from build123d import *

# Parameters (mm, degrees)
BOSS_EXTRU_1_DEPTH      = 3
ENL_V_MAT_EXTRU_1_REACH = 5
ESQUISSE3_R             = 1.75
ESQUISSE4_W             = 52.83
ESQUISSE4_H             = 19.81
BOSS_EXTRU_2_DEPTH      = 2
ESQUISSE6_W             = 6.35
ESQUISSE6_H             = 19.81
BOSS_EXTRU_3_DEPTH      = 9.74
ENL_V_START             = -6
ESQUISSE5_R             = 2.286
ENL_V_MAT_EXTRU_2_DEPTH = 16.74
ESQUISSE7_R             = 4
ENL_V_MAT_EXTRU_3_DEPTH = 6
ESQUISSE8_W             = 1
ESQUISSE8_H             = 2
ENL_V_MAT_EXTRU_4_DEPTH = 53.83
ESQUISSE9_W             = 10.19
ESQUISSE9_H             = 1
ENL_V_MAT_EXTRU_5_DEPTH = 32.415
CONG_1_R                = 2.54
CONG_2_R                = 2.54


with BuildPart() as part:
    # Esquisse2 → Boss.-Extru.1 (new body)
    with BuildSketch(Plane(origin=(0, 0, 0), x_dir=(1, 0, 0), z_dir=(0, 1, 0))):
        with BuildLine():
            Line((-4.999130413, 19.906752432), (-4.999130413, -20.093247568))
            ThreePointArc((-4.999130413, -20.093247568), (0.046625811, -24.999782599), (5, -20))
            Line((5, -20), (5, 20))
            ThreePointArc((5, 20), (-0.046625811, 24.999782599), (-4.999130413, 19.906752432))
        make_face()
    extrude(amount=BOSS_EXTRU_1_DEPTH)

    # Esquisse3 → Enlèv. mat.-Extru.1 (cut, up to next)
    with BuildSketch(Plane(origin=(0, 3, 0), x_dir=(1, 0, 0), z_dir=(0, 1, 0)), mode=Mode.PRIVATE) as enl_v_mat_extru_1_sk1:
        with Locations((0, 20)):
            Circle(ESQUISSE3_R)
    enl_v_mat_extru_1_tool1 = extrude(enl_v_mat_extru_1_sk1.sketch, amount=-ENL_V_MAT_EXTRU_1_REACH, mode=Mode.PRIVATE) & part.part
    add(enl_v_mat_extru_1_tool1.solids().sort_by_distance((0, 3, -20))[0], mode=Mode.SUBTRACT)
    # Esquisse3 → Enlèv. mat.-Extru.1 (cut, up to next)
    with BuildSketch(Plane(origin=(0, 3, 0), x_dir=(1, 0, 0), z_dir=(0, 1, 0)), mode=Mode.PRIVATE) as enl_v_mat_extru_1_sk2:
        with Locations((0, -20)):
            Circle(ESQUISSE3_R)
    enl_v_mat_extru_1_tool2 = extrude(enl_v_mat_extru_1_sk2.sketch, amount=-ENL_V_MAT_EXTRU_1_REACH, mode=Mode.PRIVATE) & part.part
    add(enl_v_mat_extru_1_tool2.solids().sort_by_distance((0, 3, 20))[0], mode=Mode.SUBTRACT)

    # Esquisse4 → Boss.-Extru.2 (add)
    with BuildSketch(Plane(origin=(0, 3, 0), x_dir=(1, 0, 0), z_dir=(0, 1, 0))):
        with Locations((0, -4.905)):
            Rectangle(ESQUISSE4_W, ESQUISSE4_H)
    extrude(amount=BOSS_EXTRU_2_DEPTH)

    # Esquisse6 → Boss.-Extru.3 (add)
    with BuildSketch(Plane(origin=(0, 5, 0), x_dir=(1, 0, 0), z_dir=(0, 1, 0))):
        with Locations((-23.24, -4.905)):
            Rectangle(ESQUISSE6_W, ESQUISSE6_H)
    boss_extru_3 = extrude(amount=BOSS_EXTRU_3_DEPTH)

    # Esquisse5 → Enlèv. mat.-Extru.2 (cut)
    with BuildSketch(Plane(origin=(0, 5, 0), x_dir=(1, 0, 0), z_dir=(0, 1, 0)).offset(ENL_V_START)):
        with Locations((-23.621, 0.174)):
            Circle(ESQUISSE5_R)
        with Locations((-23.621, -9.984)):
            Circle(ESQUISSE5_R)
    enl_v_mat_extru_2 = extrude(amount=ENL_V_MAT_EXTRU_2_DEPTH, mode=Mode.SUBTRACT)

    # Symétrie1: Boss.-Extru.3, Enlèv. mat.-Extru.2 across plane
    add(boss_extru_3.mirror(Plane(origin=(0, 0, 0), x_dir=(0, 0, 1), z_dir=(1, 0, 0))))
    add(enl_v_mat_extru_2.mirror(Plane(origin=(0, 0, 0), x_dir=(0, 0, 1), z_dir=(1, 0, 0))), mode=Mode.SUBTRACT)

    # Esquisse7 → Enlèv. mat.-Extru.3 (cut, through all)
    with BuildSketch(Plane(origin=(0, 5, 0), x_dir=(1, 0, 0), z_dir=(0, 1, 0))):
        with Locations((10.415, -4.824151883)):
            Circle(ESQUISSE7_R)
    extrude(amount=-ENL_V_MAT_EXTRU_3_DEPTH, mode=Mode.SUBTRACT)

    # Esquisse8 → Enlèv. mat.-Extru.4 (cut, through all)
    with BuildSketch(Plane(origin=(26.415, 0, 0), x_dir=(0, 0, -1), z_dir=(1, 0, 0))):
        with Locations((-4.905, 13.74)):
            Rectangle(ESQUISSE8_W, ESQUISSE8_H)
    extrude(amount=-ENL_V_MAT_EXTRU_4_DEPTH, mode=Mode.SUBTRACT)

    # Esquisse9 → Enlèv. mat.-Extru.5 (cut, through all)
    with BuildSketch(Plane(origin=(5, 0, 0), x_dir=(0, 0, -1), z_dir=(1, 0, 0))):
        with Locations((-19.905, 2.5)):
            Rectangle(ESQUISSE9_W, ESQUISSE9_H)
    extrude(amount=-ENL_V_MAT_EXTRU_5_DEPTH, mode=Mode.SUBTRACT)

    # Congé1
    cong_1_edges = [part.edges().sort_by_distance(p)[0] for p in [
        (-26.415, 8.87, -5),
        (-26.415, 8.87, 14.81),
        (26.415, 8.87, 14.81),
        (26.415, 8.87, -5),
    ]]
    fillet(cong_1_edges, radius=CONG_1_R)

    # Congé2
    cong_2_edges = [part.edges().sort_by_distance(p)[0] for p in [
        (-20.065, 9.87, 14.81),
        (-20.065, 9.87, -5),
        (20.065, 9.87, -5),
        (20.065, 9.87, 14.81),
    ]]
    fillet(cong_2_edges, radius=CONG_2_R)


solid = part.part
Input: part model. Units: mm. Frame: model coordinates. A direction names the side the tool comes from. Round coordinates to 2 decimals unless told otherwise and drop trailing zeros. Write each loop counter-clockwise with the first axis right and the second up, starting at its lowest first coordinate (ties: lowest second). Pieces come first, ordered by that corner, then holes.
1) Cut plane D-D (x = -17). Return the cut outline in (y, z).
2) Draft query along X for faces 1 (the flat face through (21, 14.74, 0)), 2 (the cylindrical face through (-21.51, 8.79, 10.86)), 3 (the flat face through (5, 1, 0)), 4 (the cylindrical face through (20.829, 9.938, -4.276)). Return one class per face: pulls with the +X half, pulls with the -X half, needs draft (parallel to the pull), parting line crosses it, or undercut.
3) Contact query for flat-ended pins moving along their axis: P1, Ø4.5, axis at x = 0, z = 20, coming from the +Y side; P2, Ø1.6, axis at x = -22.5, y = 13.5, coming from the +Z side; P3, Ø0.9, axis at y = 2, z = -3, coming from the +X side; P4, Ø2, axis at x = 18, y = 6.5, coming from the +Z side. Output: stop coordinate, or through.
4) Cut plane A-A (x = 0). Return the cut outline in (y, z).
5) Ray query, L1, parallel to X at y = 10, z = 0 (3 decimals); L2, parallel to X at y = 14.25, z = 9 (3 decimals); L3, parallel to X at y = 1.75, z = -15. Return the intervals inside material, ascending.
6) Reachability of faces 5 (the flat face through (23, 14, 5.405)), 6 (the flat face through (-4.999, 1, 0)), 7 (the flat face through (-20.065, 10, 5)) from +Z, -Z, +X, -X, +Y, -Y: full face, straight path, thin tool, end or side. Return the list, or none.
7) Cut plane C-C (z = 16.5). Return the cut outline in (x, y).
8) Cut plane B-B (x = 10.5). Return the cut outline in (y, z), then the cut area to 3 significant figures.
Geometry says:
1. outline: (3, -5) - (5, -5) - (5, 14.81) - (3, 14.81) - close
2. face 1: needs draft
2. face 2: undercut
2. face 3: pulls with the +X half
2. face 4: undercut
3. P1: stops at y = 2
3. P2: stops at z = 14.81
3. P3: stops at x = 5
3. P4: passes through
4. outline: (0, -25) - (3, -25) - (3, -21.75) - (0, -21.75) - close; (0, -18.25) - (3, -18.25) - (3, -5) - (5, -5) - (5, 14.81) - (2, 14.81) - (2, 18.25) - (0, 18.25) - close; (0, 21.75) - (2, 21.75) - (2, 25) - (0, 25) - close
5. L1: x = -26.415 to -25.9, -21.342 to -20.065, 20.065 to 21.342, 25.9 to 26.415
5. L2: x = -26.415 to -25.684, -21.558 to -20.065, 20.065 to 21.558, 25.684 to 26.415
5. L3: x = -5 to 5
6. face 5: +X, -X, +Y
6. face 6: +Z, -Z, -X, -Y
6. face 7: +Z, -Z, +Y
7. outline: (-5, 0) - (5, 0) - (5, 2) - (-5, 2) - close
8. outline: (3, -5) - (5, -5) - (5, 0.83) - (3, 0.83) - close; (3, 8.82) - (5, 8.82) - (5, 14.81) - (3, 14.81) - close
8. area: 23.6 mm2
